CAD build for the part. Positions are in the model's coordinates, mm. Give positions to 0.01 mm unless a question says otherwise; leave off trailing zeros. Order: outer loops, then holes, each group sorted by start corner. A loop starts at its lowest first (then second) coordinate and runs counter-clockwise, first axis right, second up.
```python
from build123d import *

# Parameters (mm, degrees)
EXTRUDE_THIN1_DEPTH = 6


with BuildPart() as part:
    # Sketch1 → Extrude-Thin1 (new body)
    with BuildSketch(Plane.XZ.offset(-506)):
        with BuildLine():
            Line((-21.192485275, -17.077366054), (159.500009042, -17.077366054))
            ThreePointArc((159.500009042, -17.077366054), (165.46311011, -19.520021284), (167.998964116, -25.444089427))
            Line((167.998964116, -25.444089427), (170.498955066, -184.866722883))
            ThreePointArc((170.498955066, -184.866722883), (168.057344942, -190.963100892), (162, -193.5))
            Line((162, -193.5), (-162, -193.5))
            ThreePointArc((-162, -193.5), (-167.994478635, -191.026294541), (-170.499880912, -185.044994328))
            Line((-170.499880912, -185.044994328), (-172.649915938, 221.118239298))
            ThreePointArc((-172.649915938, 221.118239298), (-166.598052627, 227.149775118), (-160.651533501, 221.014354663))
            Line((-160.651533501, 221.014354663), (-165.998338708, -15.430425982))
            ThreePointArc((-165.998338708, -15.430425982), (-164.147858351, -20.121318086), (-159.5, -22.077375097))
            Line((-159.5, -22.077375097), (-45.192485275, -22.077375097))
            Line((-45.192485275, -22.077375097), (-45.192485275, -24.077375097))
            Line((-45.192485275, -24.077375097), (-159.499998361, -24.077375097))
            ThreePointArc((-159.499998361, -24.077375097), (-165.577967625, -21.519455227), (-167.997827562, -15.385211808))
            Line((-167.997827562, -15.385211808), (-162.651022334, 221.059569775))
            ThreePointArc((-162.651022334, 221.059569775), (-166.615368418, 225.149850079), (-170.649943958, 221.128826199))
            Line((-170.649943958, 221.128826199), (-168.499908932, -185.034407427))
            ThreePointArc((-168.499908932, -185.034407427), (-166.584013074, -189.608342884), (-162, -191.5))
            Line((-162, -191.5), (162, -191.5))
            ThreePointArc((162, -191.5), (166.632088112, -189.560017513), (168.499200897, -184.898079914))
            Line((168.499200897, -184.898079914), (165.999209981, -25.475448634))
            ThreePointArc((165.999209981, -25.475448634), (164.060027506, -20.945278877), (159.500009042, -19.077366054))
            Line((159.500009042, -19.077366054), (-21.192485275, -19.077366054))
            Line((-21.192485275, -19.077366054), (-21.192485275, -17.077366054))
        make_face()
    extrude(amount=EXTRUDE_THIN1_DEPTH)


solid = part.part
```
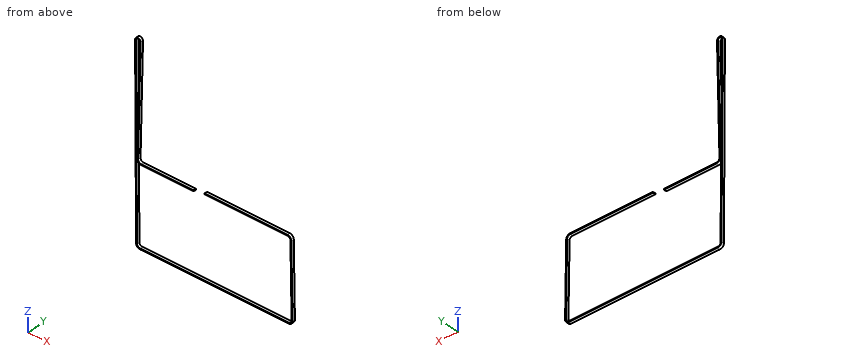
Item 1: Slice it at B-B (y = 501.15). Give the cut face in (x, z) (3 decimals).
Item 2: Wall check: L1, parallel to Z at x = -17, y = 504.6; L2, parallel to Z at x = -114, y = 500.9; L3, parallel to X at y = 502.6, z = 7.5. Give the ranges that are in metal, low to high.
Item 3: Slice it at A-A (x = 0). Give the cut face in (y, z).
Item 4: Drop flat-ended pins along their axis: pin 1 Ø3 at (x, y) = (26.5, 503.5) entering from +Z; pin 2 Ø1 at (y, z) = (503, -18.5) entering from -X; pin 3 Ø1.8 at (x, y) = (-97.5, 502) entering from +Z. Give the stop position or say it passes through.
Item 5: Slice it at C-C (z = -152.5). Give the cut face in (x, y), and give its area (3 significant figures).
A:
1. outline: (-172.65, 221.118) - (-170.5, -185.045) arc R8.5 ccw to (-162, -193.5) - (162, -193.5) arc R8.5 ccw to (170.499, -184.867) - (167.999, -25.444) arc R8.5 ccw to (159.5, -17.077) - (-21.192, -17.077) - (-21.192, -19.077) - (159.5, -19.077) arc R6.5 cw to (165.999, -25.475) - (168.499, -184.898) arc R6.5 cw to (162, -191.5) - (-162, -191.5) arc R6.5 cw to (-168.5, -185.034) - (-170.65, 221.129) arc R4 cw (long way) to (-162.651, 221.06) - (-167.998, -15.385) arc R8.5 ccw to (-159.5, -24.077) - (-45.192, -24.077) - (-45.192, -22.077) - (-159.5, -22.077) arc R6.5 cw to (-165.998, -15.43) - (-160.652, 221.014) arc R6 ccw (long way) to start
2. L1: z = -193.5 to -191.5, -19.08 to -17.08
2. L2: z = -193.5 to -191.5, -24.08 to -22.08
2. L3: x = -171.52 to -169.52, -167.48 to -165.48
3. outline: (500, -193.5) - (506, -193.5) - (506, -191.5) - (500, -191.5) - close; (500, -19.08) - (506, -19.08) - (506, -17.08) - (500, -17.08) - close
4. pin 1: stops at z = -17.08
4. pin 2: stops at x = -171.38
4. pin 3: stops at z = -22.08
5. outline: (-170.67, 500) - (-168.67, 500) - (-168.67, 506) - (-170.67, 506) - close; (167.99, 500) - (169.99, 500) - (169.99, 506) - (167.99, 506) - close
5. area: 24.0 mm2
